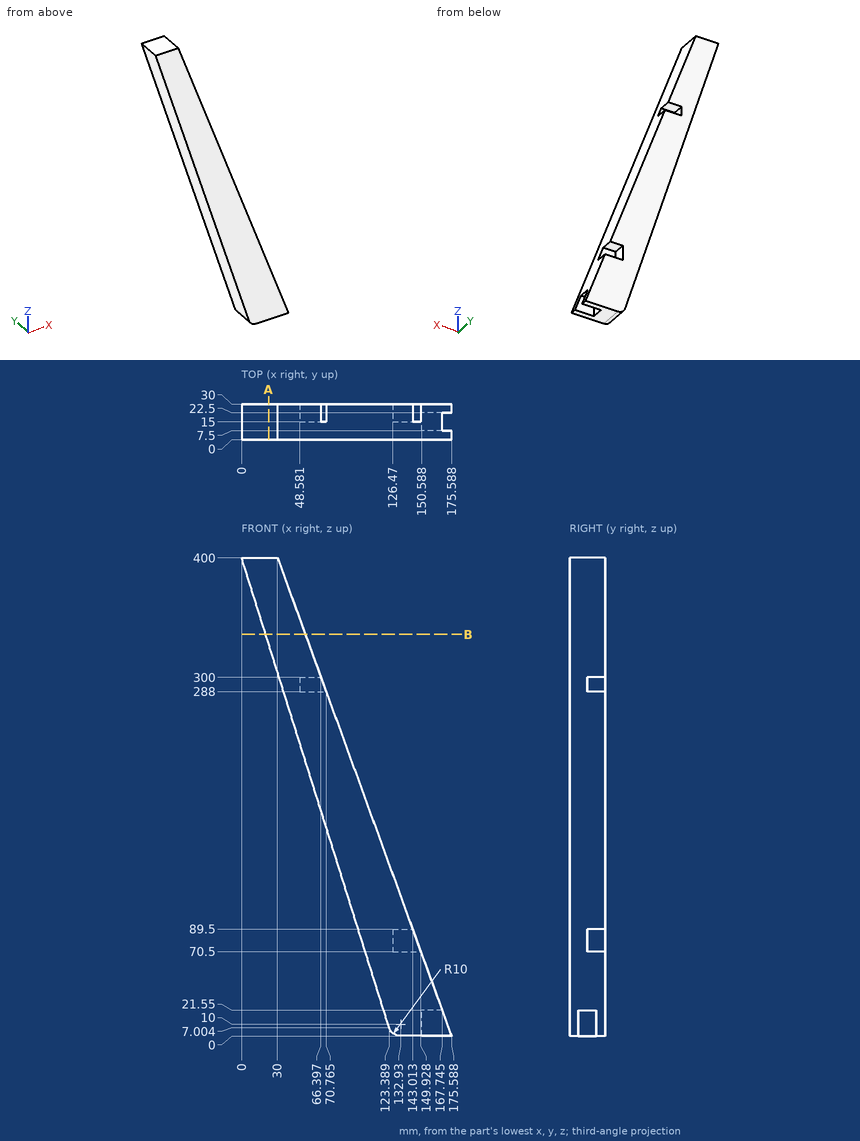
Design review of the part shown in the three views and the two pictorial views. Dimensions are in mm from the part's minimum x, y and z. Give positions to 0.01 mm unless a question says otherwise; leave off trailing zeros. Write each loop counter-clockwise with the first axis right and the second up, starting at its lowest first coordinate (ties: lowest second). Pieces come first, ordered by that corner, then holes.
(1) Wall thickness on line 1 along X through (y, z) = (18.5, 245.5) (1 decimal); line 2 along X through (y, z) = (19.5, 322.5): over which ranges is each line inside the solid? List them lowest first.
Checked values:
line 1: x = 48.5 to 86.2
line 2: x = 24.33 to 58.21
(2) Add section B-B (z = 336). Give the boundary of the cut face in (x, y) (1 decimal).
Checked values:
outline: (20.1, 0) - (53.3, 0) - (53.3, 30) - (20.1, 30) - close
(3) Clearance check with flat-ended pins moving along their axes: pin 1 Ø12 at (y, z) = (21.5, 100) entering from +X (1 decimal); pin 2 Ø2 at (y, z) = (24.5, 189.5) entering from -X; pin 3 Ø5 at (y, z) = (10.5, 54.5) entering from -X. State where each tip first meets the part, or that it passes through.
Checked values:
pin 1: stops at x = 141.4
pin 2: stops at x = 65.78
pin 3: stops at x = 107.69
(4) Add section A-A (x = 22.5). Give the boundary of the cut face in (y, z), and give its area (3 significant figures).
Checked values:
outline: (0, 328.34) - (30, 328.34) - (30, 400) - (0, 400) - close
area: 2,150 mm2
